Check sheet for the modelled part. Datum: model origin and axes. Units: mm. Round coordinates to 2 decimals unless told otherwise and drop trailing zeros. Loops run counter-clockwise (first coordinate to the right, second up) from the corner with the lowest first, then second, coordinate; pieces in that order, holes last. Notation, with made-up numbers: (-37.75, -33) - (-25.75, -33) arc R18 cw to (-25.75, -8) - close; hole circle Ø2 at (2, 78). An arc over 180 degrees is marked (long way). Return JSON: item names as keys, results as strings.
from build123d import *

# Parameters (mm, degrees)
SKETCH1_R           = 2.5
BOSS_EXTRUDE1_DEPTH = 5.08
FILLET1_R           = 5.08
FILLET2_R           = 5.08
CUT_EXTRUDE1_DEPTH  = 6.08


with BuildPart() as part:
    # Sketch1 → Boss-Extrude1 (new body)
    with BuildSketch(Plane(origin=(0, 0, 0), x_dir=(1, 0, 0), z_dir=(0, 1, 0))):
        Polygon((0, 0), (0, 76.2), (25.4, 76.2), (76.2, 25.4), (76.2, 0), align=None)
        with Locations((12.7, 63.5)):
            Circle(SKETCH1_R, mode=Mode.SUBTRACT)
        with Locations((63.5, 12.7)):
            Circle(SKETCH1_R, mode=Mode.SUBTRACT)
        with Locations((12.7, 46.99)):
            Circle(SKETCH1_R, mode=Mode.SUBTRACT)
        with Locations((12.7, 30.48)):
            Circle(SKETCH1_R, mode=Mode.SUBTRACT)
        with Locations((46.99, 12.7)):
            Circle(SKETCH1_R, mode=Mode.SUBTRACT)
        with Locations((30.48, 12.7)):
            Circle(SKETCH1_R, mode=Mode.SUBTRACT)
        with Locations((12.7, 12.7)):
            Circle(SKETCH1_R, mode=Mode.SUBTRACT)
    extrude(amount=BOSS_EXTRUDE1_DEPTH)

    # Fillet1
    fillet1_edges = [part.edges().sort_by_distance(p)[0] for p in [
        (0, 2.54, 0),
    ]]
    fillet(fillet1_edges, radius=FILLET1_R)

    # Fillet2
    fillet2_edges = [part.edges().sort_by_distance(p)[0] for p in [
        (0, 2.54, -76.2),
        (25.4, 2.54, -76.2),
        (76.2, 2.54, -25.4),
        (76.2, 2.54, 0),
    ]]
    fillet(fillet2_edges, radius=FILLET2_R)

    # Sketch2 → Cut-Extrude1 (cut, through all)
    with BuildSketch(Plane(origin=(0, 5.08, 0), x_dir=(1, 0, 0), z_dir=(0, 1, 0))):
        with BuildLine():
            Line((18.765620134, 62.732842611), (62.732842611, 18.765620134))
            ThreePointArc((62.732842611, 18.765620134), (62.746984747, 18.765620134), (62.746984747, 18.77976227))
            Line((62.746984747, 18.77976227), (18.77976227, 62.746984747))
            ThreePointArc((18.77976227, 62.746984747), (18.765620134, 62.746984747), (18.765620134, 62.732842611))
        make_face()
        with BuildLine():
            Line((18.763824083, 41.796641641), (41.796641641, 18.763824083))
            ThreePointArc((41.796641641, 18.763824083), (41.800233744, 18.763824083), (41.800233744, 18.767416186))
            Line((41.800233744, 18.767416186), (18.767416186, 41.800233744))
            ThreePointArc((18.767416186, 41.800233744), (18.763824083, 41.800233744), (18.763824083, 41.796641641))
        make_face()
        with BuildLine():
            Line((24.444358625, 18.548492515), (18.548492515, 24.444358625))
            ThreePointArc((18.548492515, 24.444358625), (18.544900412, 24.444358625), (18.544900412, 24.440766523))
            Line((18.544900412, 24.440766523), (24.440766523, 18.544900412))
            ThreePointArc((24.440766523, 18.544900412), (24.444358625, 18.544900412), (24.444358625, 18.548492515))
        make_face()
    extrude(amount=-CUT_EXTRUDE1_DEPTH, mode=Mode.SUBTRACT)

    # Mirror1: part across plane


with BuildPart() as part_1:
    add(part.part)
    add(part.part.mirror(Plane.XY.offset(-12.7)))


solid = part_1.part
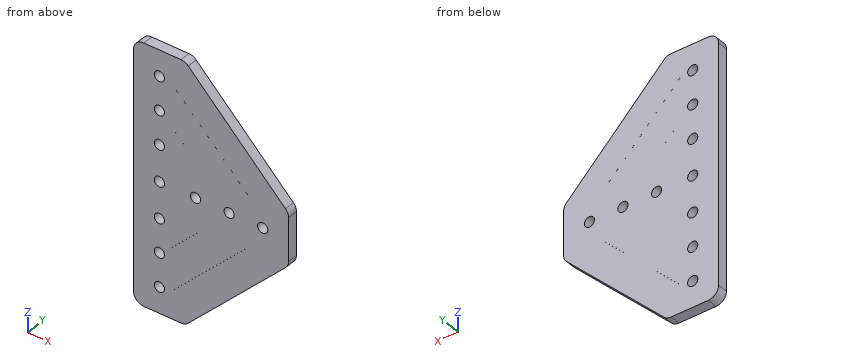
Q1. Scan lines: probe 1 along Z at (x, y) = (63.5, 3.25); probe 2 along Z at (x, y) = (65.5, 1.55). Record each from-to range of solid material in increasing order. Write a range as [from, to].
Answer key:
{"probe 1": "z = [-38.1, -15.2], [-10.2, 12.7]", "probe 2": "z = [-36.1, -14.2], [-11.2, 10.7]"}
Q2. Sectioned sample at B-B (z = -30.48). Enter the section's corners in (x, y), plus the area to 3 significant figures.
Answer key:
{"outline": "(0, 0) - (10.2, 0) - (10.2, 5.08) - (0, 5.08) - close; (15.2, 0) - (30.08, 0) - (30.08, 5.08) - (15.2, 5.08) - close; (30.09, 0) - (51.02, 0) - (51.02, 5.08) - (30.09, 5.08) - close; (51.05, 0) - (71.12, 0) - (71.12, 5.08) - (51.05, 5.08) - close", "area": "336 mm²"}
Q3. Depth check by flat-ended pin: P1, Ø6.5, axis at x = 30.48, z = -12.7, coming from the -Y side. Enter the tip coordinate at first touch or a pass-through.
Answer key:
{"P1": "stops at y = 0"}
Q4. Sectioned sample at A-A (x = 12.7). State how many separate pieces and enclosed holes the cut face has, plus the area to 3 significant figures.
Answer key:
{"separate pieces": "8", "enclosed holes": "0", "area": "467 mm²"}
Q5. Sectioned sample at C-C (z = 26.5). Enter the section's corners in (x, y), plus the area to 3 significant figures.
Answer key:
{"outline": "(0, 0) - (29.6, 0) - (29.6, 5.08) - (0, 5.08) - close; (29.63, 0) - (49.7, 0) - (49.7, 5.08) - (29.63, 5.08) - close", "area": "252 mm²"}
